Here's how the part is built. I have some questions about the finished solid (model axes, mm). A direction names the side the tool comes from. Round coordinates to 2 decimals unless told otherwise and drop trailing zeros. Loops run counter-clockwise (first coordinate to the right, second up) from the corner with the lowest first, then second, coordinate; pieces in that order, holes last. Notation, with made-up numbers: M 27,50.5 L 54,50.5 A36 ccw 54,86.5 Z; hole C 77,-12.5 d4. An arc over 180 degrees is marked long. Answer as a JSON object with one key per item and string values.
from build123d import *

# Parameters (mm, degrees)
SKETCH1_W           = 228.6
SKETCH1_H           = 76.2
BOSS_EXTRUDE1_DEPTH = 25.4
SKETCH2_R           = 7.62
SKETCH2_W           = 25.4
SKETCH2_H           = 12.7
BOSS_EXTRUDE2_DEPTH = 254


with BuildPart() as part:
    # Sketch1 → Boss-Extrude1 (new body)
    with BuildSketch(Plane(origin=(0, 0, 0), x_dir=(1, 0, 0), z_dir=(0, 1, 0))):
        with Locations((0, 26.13343465)):
            Rectangle(SKETCH1_W, SKETCH1_H)
    extrude(amount=BOSS_EXTRUDE1_DEPTH)

    # Sketch2 → Boss-Extrude2 (add)
    with BuildSketch(Plane(origin=(0, 25.4, 0), x_dir=(1, 0, 0), z_dir=(0, 1, 0))):
        with Locations(Location((-101.6, 0, 0), (0, 0, 90))):
            Circle(SKETCH2_R)
        with Locations(Location((101.6, -0.915640228, 0), (0, 0, 90))):
            Circle(SKETCH2_R)
        with Locations((0, 50.068949407)):
            Rectangle(SKETCH2_W, SKETCH2_H)
    extrude(amount=BOSS_EXTRUDE2_DEPTH)


solid = part.part
Item 1: I want a section at C-C, the plane z = -0.5. Please give me the cut outline in (x, y), then the cut area to 3 significant figures.
Resolved:
{"outline": "M -114.3,0 L 114.3,0 L 114.3,25.4 L 109.09,25.4 L 109.09,279.4 L 94.11,279.4 L 94.11,25.4 L -94,25.4 L -94,279.4 L -109.2,279.4 L -109.2,25.4 L -114.3,25.4 Z", "area": "13,500 mm²"}
Item 2: On a 3-axis mill with a long thin cutter (end or side, diameter ignored), from which of +Z, -Z, +X, -X, +Y, -Y can I reach the whole of each face in a straight line? I mean faces 1 (the face through (12.7, 151, -50)), 2 (the face through (-12.7, 151, -50)), 3 (the face through (-109.155, 150.622, 0.992)), 4 (the face through (0, 151, -43.719)). Say none if no direction works.
Resolved:
{"face 1": "+Z, -Z, +X, +Y", "face 2": "+Z, -Z, -X, +Y", "face 3": "+Y", "face 4": "+Z, +X, -X, +Y"}
Item 3: Please list where these lines run through material, in increasing order: probe 1 along Y at (x, z) = (78, -12); probe 2 along Z at (x, y) = (-12, 211.5); probe 3 along X at (y, z) = (78.5, -44). Write a range as from..to.
Resolved:
{"probe 1": "0..25.4", "probe 2": "-56.42..-43.72", "probe 3": "-12.7..12.7"}
Item 4: I'm going to push flat-ended pins straight in: pin 1 Ø12 at (y, z) = (73.5, -37.5) entering from -X; pin 2 Ø1.5 at (y, z) = (124.5, -45.5) entering from -X; pin 3 Ø8 at (x, z) = (62.5, -14.5) entering from +Y; pin 4 Ø10 at (x, z) = (-68, -45.5) entering from -Y. Where does each tip first touch, or does it pass through?
Resolved:
{"pin 1": "through", "pin 2": "x = -12.7", "pin 3": "y = 25.4", "pin 4": "y = 0"}
Item 5: I want a section at B-B, the plane x = -101.6. Please give me the cut outline in (y, z), then the cut area to 3 significant figures.
Resolved:
{"outline": "M 0,-64.23 L 25.4,-64.23 L 25.4,-7.62 L 279.4,-7.62 L 279.4,7.62 L 25.4,7.62 L 25.4,11.97 L 0,11.97 Z", "area": "5,810 mm²"}
Item 6: I want a section at A-A, the plane y = 60. Please give me the cut outline in (x, z), then the cut area to 3 significant figures.
Resolved:
{"outline": "C -101.6,0 d15.24; M -12.7,-56.42 L 12.7,-56.42 L 12.7,-43.72 L -12.7,-43.72 Z; C 101.6,0.92 d15.24", "area": "687 mm²"}
Item 7: I want a section at D-D, the plane x = -6. Please give me the cut outline in (y, z), then the cut area to 3 significant figures.
Resolved:
{"outline": "M 0,-64.23 L 25.4,-64.23 L 25.4,-56.42 L 279.4,-56.42 L 279.4,-43.72 L 25.4,-43.72 L 25.4,11.97 L 0,11.97 Z", "area": "5,160 mm²"}
